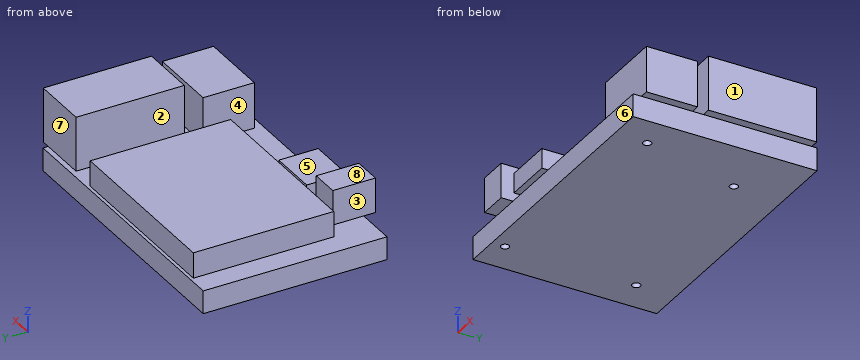
```python
from build123d import *

# Parameters (mm, degrees)
F0_W     = 85
F0_H     = 56
F1_DEPTH = 7
F2_W     = 14.75
F2_H     = 33
F2_W_2   = 2.65
F3_DEPTH = 16.6
F2_W_3   = 18.95
F2_H_2   = 15.6
F4_DEPTH = 14
F2_W_4   = 14.8
F2_H_3   = 10.1
F2_H_4   = 1.9
F5_DEPTH = 6
F2_W_5   = 8.8
F2_H_5   = 9.4
F2_H_6   = 3.6
F6_DEPTH = 10.6
F2_W_6   = 54.7
F2_H_7   = 42.8
F7_DEPTH = 7.8
F8_D     = 2.5
F8_DEPTH = 5
F8_TIP   = 0.7510757738


with BuildPart() as f1:
    # F0 (on Top) → F1 (new body)
    with BuildSketch(Plane.XY):
        Rectangle(F0_W, F0_H)
    extrude(amount=F1_DEPTH)

    # F2 (on face) → F3 (join)
    with BuildSketch(Plane.XY.offset(7)):
        with Locations((35.125, 9.9)):
            Rectangle(F2_W, F2_H)
        with Locations((43.825, 9.9)):
            Rectangle(F2_W_2, F2_H)
    extrude(amount=F3_DEPTH)

    # F2 (on face) → F4 (join)
    with BuildSketch(Plane.XY.offset(7)):
        with Locations((33.025, -17.7)):
            Rectangle(F2_W_3, F2_H_2)
        with Locations((43.825, -17.7)):
            Rectangle(F2_W_2, F2_H_2)
    extrude(amount=F4_DEPTH)

    # F2 (on face) → F5 (join)
    with BuildSketch(Plane.XY.offset(7)):
        with Locations((-10.1, -22.95)):
            Rectangle(F2_W_4, F2_H_3)
        with Locations((-10.1, -28.95)):
            Rectangle(F2_W_4, F2_H_4)
    extrude(amount=F5_DEPTH)

    # F2 (on face) → F6 (join)
    with BuildSketch(Plane.XY.offset(7)):
        with Locations((-25.7, -23.3)):
            Rectangle(F2_W_5, F2_H_5)
        with Locations((-25.7, -29.8)):
            Rectangle(F2_W_5, F2_H_6)
    extrude(amount=F6_DEPTH)

    # F2 (on face) → F7 (join)
    with BuildSketch(Plane.XY.offset(7)):
        with Locations((-8.15, 5.6)):
            Rectangle(F2_W_6, F2_H_7)
    extrude(amount=F7_DEPTH)

    # F8
    with Locations(Plane(origin=(0, 0, 0), x_dir=(1, 0, 0), z_dir=(0, 0, -1))):
        with Locations((-32.5, 24), (32.5, 18), (24.5, -13), (-32.5, -16)):
            Hole(F8_D / 2, depth=F8_DEPTH)
            with Locations((0, 0, -(F8_DEPTH + F8_TIP / 2))):  # 118° drill point
                Cone(0, F8_D / 2, F8_TIP, mode=Mode.SUBTRACT)


solid = f1.part
```
Check sheet for the modelled part. Datum: model origin and axes. Units: mm. Face numbers are marked on the shaded views. A direction names the side the tool comes from. Coordinates: 2 decimals unless noted, no trailing zeros. Write each loop counter-clockwise with the first axis right and the second up, starting at its lowest first coordinate (ties: lowest second). Pieces come first, ordered by that corner, then holes. Notation, with made-up numbers: M 44.25,-40 L 70.25,-40 A19 ccw 70.25,-7 Z; hole C 13,83 d7. An arc over 180 degrees is marked long. Write item = value, one per line. Start each with the question number.
1. Thickness scan on probe 1 along Y at (x, z) = (-32.5, 2.5); probe 2 along Y at (x, z) = (-28, 11.25); probe 3 along X at (y, z) = (-18, 12.25). Record the ranges inside material, lowest first.
2. Sectioned sample at A-A (z = 16.25). Record the cut outline in (x, y).
3. Mould release check, pull along X, two halves, no side actions. Record for the marked faces 1, 2 and 3: pulls with the +X half, pulls with the -X half, needs draft (parallel to the pull), parting line crosses it, or undercut.
4. Sectioned sample at D-D (x = -12.5). Record the cut outline in (y, z).
5. Sectioned sample at B-B (x = 17). Record the cut outline in (y, z).
6. Sectioned sample at C-C (y = -14). Record the cut outline in (x, z), then the cut area to 3 significant figures.
7. Tool access check on the marked faces 4, 5, 6, 7 and 8. Record the directions out of +Z, -Z, +X, -X, +Y, -Y that give a thin tool (end or side, any length) a straight path to the whole face; none if there is none.
8. Go/stop test with flat-tipped pins: pin 1 (7 mm diameter, centred on y = -21.5, z = 12, fed in from -X); pin 2 (2 mm diameter, centred on y = 8, z = 2, fed in from +X); pin 3 (1 mm diameter, centred on x = 17, y = 0, fed in from -Z); pin 4 (1.5 mm diameter, centred on x = -7, z = 11.5, fed in from -Y). Record where each tip stops, or that it passes through.
The answers:
q1.probe_1 = -28 to -25.25, -22.75 to 14.75, 17.25 to 28
q1.probe_2 = -31.6 to -18.6, -15.8 to 27
q1.probe_3 = -17.5 to -2.7, 23.55 to 45.15
q2.outline = M -30.1,-31.6 L -21.3,-31.6 L -21.3,-18.6 L -30.1,-18.6 Z; M 23.55,-25.5 L 45.15,-25.5 L 45.15,-9.9 L 23.55,-9.9 Z; M 27.75,-6.6 L 45.15,-6.6 L 45.15,26.4 L 27.75,26.4 Z
q3.face_1 = pulls with the +X half
q3.face_2 = undercut
q3.face_3 = pulls with the -X half
q4.outline = M -29.9,7 L -28,7 L -28,0 L 28,0 L 28,7 L 27,7 L 27,14.8 L -15.8,14.8 L -15.8,7 L -17.9,7 L -17.9,13 L -29.9,13 Z
q5.outline = M -28,0 L 28,0 L 28,7 L 27,7 L 27,14.8 L -15.8,14.8 L -15.8,7 L -28,7 Z
q6.outline = M -42.5,0 L 42.5,0 L 42.5,7 L 45.15,7 L 45.15,21 L 23.55,21 L 23.55,7 L 19.2,7 L 19.2,14.8 L -35.5,14.8 L -35.5,7 L -42.5,7 Z
q6.area = 1,320 mm²
q7.face_4 = +Z, +Y, -Y
q7.face_5 = +Z, -Y
q7.face_6 = -Z, +X, -X, -Y
q7.face_7 = +Z, +X, +Y
q7.face_8 = +Z, -X, +Y, -Y
q8.pin_1 = -30.1
q8.pin_2 = 42.5
q8.pin_3 = 0
q8.pin_4 = -29.9
